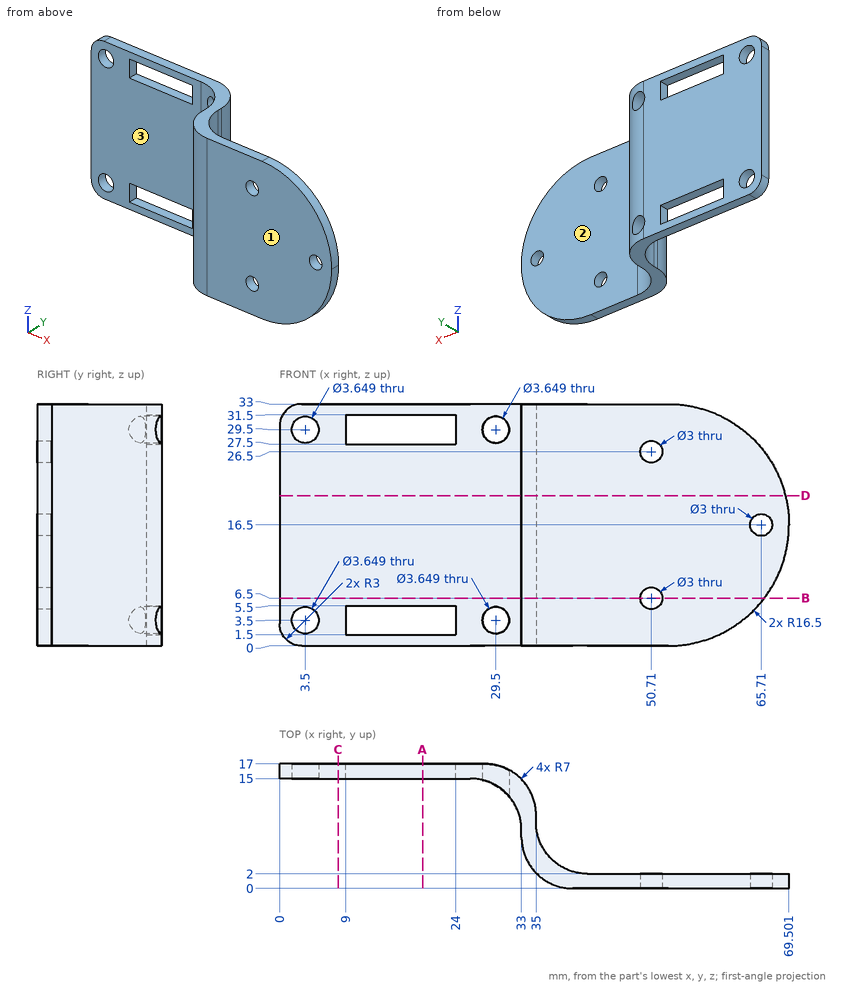
For this review, use the dimensioned drawing (mm, ordinates from the lowest corner) and the shaded views. A direction names the side the tool comes from. Round coordinates to 2 decimals unless told otherwise and drop trailing zeros. Write each loop counter-clockwise with the first axis right and the second up, starting at its lowest first coordinate (ties: lowest second). Pieces come first, ordered by that corner, then holes. Notation, with made-up numbers: (20.25, 14) - (54.25, 14) arc R19 cw to (54.25, 40) - close; hole circle Ø7 at (20, -40). An arc over 180 degrees is marked (long way). Answer as CSV lines item,"result". Start each with the question number.
(1) To check wall thickness, follow line 1 (X direction, y = 16.3, z = 29.5) (1 decimal); line 2 (Y direction, x = 7, z = 30); line 3 (Y direction, x = 52, z = 13.5). State the ranges of each line that lie inside material, in increasing order.
(2) We need section A-A on x = 19.5. State the section outline as (y, z) points, plus the area to 3 significant figures.
(3) We need section B-B on z = 6.5. State the section outline as (x, y) points.
(4) For the marked faces 1, 2 and 3, list the 3-axis set-ups (+Z, -Z, +X, -X, +Y, -Y) from which the entire face can be reached by the end or side of a thin tool; tool diameter is ignored.
(5) For pin 1 Ø6 at (x, z) = (3.5, 29.5) entering from -Y; pin 2 Ø14 at (x, z) = (49.5, 17.5) entering from +Y; pin 3 Ø1.6 at (y, z) = (16.5, 29.5) entering from +X (1 decimal), all flat-tipped, find the tip position at first contact; note any pin that passes through.
(6) We need section C-C on x = 8. State the section outline as (y, z) points, plus the area to 3 significant figures.
(7) We need section D-D on z = 20.5. State the section outline as (x, y) points.
Worked answers:
1,line 1,"0 to 1.7, 5.3 to 9, 24 to 27.7"
1,line 2,"15 to 17"
1,line 3,"0 to 2"
2,outline,"(15, 0) - (17, 0) - (17, 1.5) - (15, 1.5) - close; (15, 5.5) - (17, 5.5) - (17, 27.5) - (15, 27.5) - close; (15, 31.5) - (17, 31.5) - (17, 33) - (15, 33) - close"
2,area,"50.0 mm²"
3,outline,"(0, 15) - (26, 15) arc R7 cw to (33, 8) - (33, 7) arc R7 ccw to (40, 0) - (49.21, 0) - (49.21, 2) - (42, 2) arc R7 cw to (35, 9) - (35, 10) arc R7 ccw to (28, 17) - (0, 17) - close; (52.21, 0) - (66.13, 0) - (66.13, 2) - (52.21, 2) - close"
4,face 1,"+Z, -Z, +X, -X, -Y"
4,face 2,"+Z, -Z, +X, +Y"
4,face 3,"+Z, -Z, -X, -Y"
5,pin 1,"y = 15"
5,pin 2,"y = 2"
5,pin 3,"x = 32.1"
6,outline,"(15, 0) - (17, 0) - (17, 33) - (15, 33) - close"
6,area,"66.0 mm²"
7,outline,"(0, 15) - (26, 15) arc R7 cw to (33, 8) - (33, 7) arc R7 ccw to (40, 0) - (69.01, 0) - (69.01, 2) - (42, 2) arc R7 cw to (35, 9) - (35, 10) arc R7 ccw to (28, 17) - (0, 17) - close"
